Verification items for the finished model (mm, model axes). Face numbers are marked on the shaded views. Round coordinates to 2 decimals unless told otherwise and drop trailing zeros. Write each loop counter-clockwise with the first axis right and the second up, starting at its lowest first coordinate (ties: lowest second). Pieces come first, ordered by that corner, then holes. Notation, with made-up numbers: M 80.5,71.25 L 107.5,71.25 A22 cw 107.5,108.25 Z; hole C 0,-35.5 d7. An arc over 180 degrees is marked long. Write each question's results on one line, items separated by ' | '.
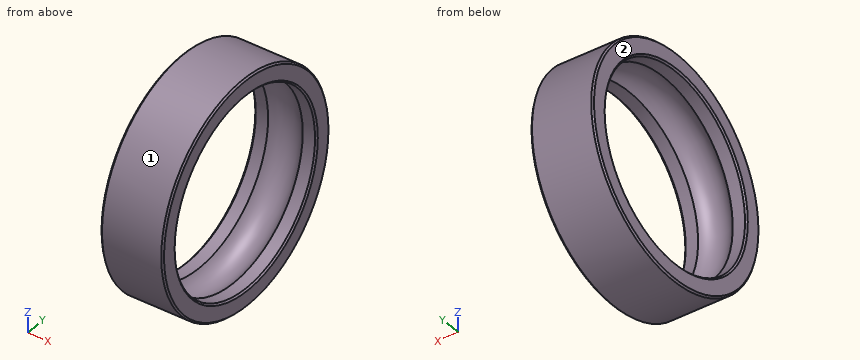
Autodesk Inventor part; units mm, degrees
ref_plane "OR_Cage_XY" through (0, 0, 0) normal (1, 0, 0) x (0, 0, -1)
ref_plane "OR_Cage_YZ" through (0, 0, 0) normal (0, 0, -1) x (0, 1, 0)
ref_plane "OR_Cage_ZX" through (0, 0, 0) normal (0, 1, 0) x (1, 0, 0)
sketch "Sketch_3" plane through (0, 0, 0) normal (0, 0, 1) x (1, 0, 0)
  line L0 (5, 0) -> (0, 0)
  line L1 (0, 8.875) -> (0, 7.725)
  line L2 (0, 7.725) -> (0.125, 7.6)
  line L3 (0.125, 7.6) -> (1.1144, 7.6)
  arc A0 (3.8856, 7.6) -> (1.1144, 7.6) centre (2.5, 6.8) ccw
  line L4 (3.8856, 7.6) -> (4.875, 7.6)
  line L5 (4.875, 7.6) -> (5, 7.725)
  line L6 (5, 7.725) -> (5, 8.875)
  line L7 (5, 8.875) -> (4.875, 9)
  line L8 (4.875, 9) -> (0.125, 9)
  line L9 (0.125, 9) -> (0, 8.875)
revolve "Revolution1" add sketch "Sketch_3" angle 360 about axis through (5, 0, 0) along (1, 0, 0)
ref_plane "OR_Cage_XY" through (0, 0, 0) normal (1, 0, 0) x (0, 0, -1)
ref_plane "OR_Cage_YZ" through (0, 0, 0) normal (0, 0, -1) x (0, 1, 0)
ref_plane "OR_Cage_ZX" through (0, 0, 0) normal (0, 1, 0) x (1, 0, 0)
ref_plane "OR_IR_XY" through (0, 0, 0) normal (1, 0, 0) x (0, 0, -1)
ref_plane "OR_IR_YZ" through (0, 0, 0) normal (0, 0, -1) x (0, 1, 0)
ref_plane "OR_IR_ZX" through (0, 0, 0) normal (0, 1, 0) x (1, 0, 0)
ref_plane "OR_ball_1_XY" through (2.5, 6.8, 0) normal (1, 0, 0) x (0, 0, -1)
ref_plane "OR_ball_1_YZ" through (2.5, 6.8, 0) normal (0, 0, -1) x (0, 1, 0)
ref_plane "OR_ball_1_ZX" through (2.5, 6.8, 0) normal (0, 1, 0) x (1, 0, 0)
ref_plane "OR_ball_2_XY" through (2.5, 3.4, 5.889) normal (1, 0, 0) x (0, 0, -1)
ref_plane "OR_ball_2_YZ" through (2.5, 3.4, 5.889) normal (0, 0, -1) x (0, 1, 0)
ref_plane "OR_ball_2_ZX" through (2.5, 3.4, 5.889) normal (0, 1, 0) x (1, 0, 0)
ref_plane "OR_ball_3_XY" through (2.5, -3.4, 5.889) normal (1, 0, 0) x (0, 0, -1)
ref_plane "OR_ball_3_YZ" through (2.5, -3.4, 5.889) normal (0, 0, -1) x (0, 1, 0)
ref_plane "OR_ball_3_ZX" through (2.5, -3.4, 5.889) normal (0, 1, 0) x (1, 0, 0)
ref_plane "OR_ball_4_XY" through (2.5, -6.8, 0) normal (1, 0, 0) x (0, 0, -1)
ref_plane "OR_ball_4_YZ" through (2.5, -6.8, 0) normal (0, 0, -1) x (0, 1, 0)
ref_plane "OR_ball_4_ZX" through (2.5, -6.8, 0) normal (0, 1, 0) x (1, 0, 0)
ref_plane "OR_ball_5_XY" through (2.5, -3.4, -5.889) normal (1, 0, 0) x (0, 0, -1)
ref_plane "OR_ball_5_YZ" through (2.5, -3.4, -5.889) normal (0, 0, -1) x (0, 1, 0)
ref_plane "OR_ball_5_ZX" through (2.5, -3.4, -5.889) normal (0, 1, 0) x (1, 0, 0)
ref_plane "OR_ball_6_XY" through (2.5, 3.4, -5.889) normal (1, 0, 0) x (0, 0, -1)
ref_plane "OR_ball_6_YZ" through (2.5, 3.4, -5.889) normal (0, 0, -1) x (0, 1, 0)
ref_plane "OR_ball_6_ZX" through (2.5, 3.4, -5.889) normal (0, 1, 0) x (1, 0, 0)
properties part number "040102DR-18-H8_or"
1) Sectioned sample at A-A, the plane y = 0. Record the cut outline in (x, z) (3 decimals), and give its area (3 significant figures).
Calculated:
outline: M 0,-8.875 L 0.125,-9 L 4.875,-9 L 5,-8.875 L 5,-7.725 L 4.875,-7.6 L 3.886,-7.6 A1.6 cw 1.114,-7.6 L 0.125,-7.6 L 0,-7.725 Z; M 0,7.725 L 0.125,7.6 L 1.114,7.6 A1.6 cw 3.886,7.6 L 4.875,7.6 L 5,7.725 L 5,8.875 L 4.875,9 L 0.125,9 L 0,8.875 Z | area: 10.8 mm²
2) Depth check by flat-ended pin: P1, Ø1, axis at x = 3, z = -4.5, coming from the +Y side; P2, Ø2, axis at y = 6.5, z = -1.5, coming from the -X side; P3, Ø1.5, axis at x = 4, z = -6, coming from the -Y side; P4, Ø2, axis at y = -5.5, z = -4.5, coming from the +X side. Enter the tip coordinate at first touch or a pass-through.
Calculated:
P1: stops at y = 8.06 | P2: stops at x = 0.05 | P3: stops at y = -7.31 | P4: stops at x = 5
3) Material ranges on line 1 (Z direction, x = 0.85, y = 0); line 2 (Y direction, x = 3.6, z = 4.75); line 3 (Y direction, x = 4.5, z = -3), recorded low to high. Write a range as [from, to].
Calculated:
line 1: z = [-9, -7.6], [7.6, 9] | line 2: y = [-7.64, -6.39], [6.39, 7.64] | line 3: y = [-8.49, -6.98], [6.98, 8.49]
4) Sectioned sample at C-C, the plane x = 0.45. Record the cut outline in (y, z), and give its area (3 significant figures).
Calculated:
outline: C 0,0 d18; hole C 0,0 d15.2 | area: 73.0 mm²
5) Draft check along Y on the marked faces 1 and 2. Enter one of: pulls with the +Y half, pulls with the -Y half, needs draft (parallel to the pull), parting line crosses it, or undercut.
Calculated:
face 1: parting line crosses it | face 2: needs draft
6) Sectioned sample at D-D, the plane x = 1.9. Record the cut outline in (y, z), and give its area (3 significant figures).
Calculated:
outline: C 0,0 d18; hole C 0,0 d16.57 | area: 38.9 mm²
